Autodesk Inventor part; units mm, degrees
ref_plane "YZ Plane" through (0, 0, 0) normal (1, 0, 0) x (0, 1, 0)
ref_plane "XZ Plane" through (0, 0, 0) normal (0, 1, 0) x (-1, 0, 0)
ref_plane "XY Plane" through (0, 0, 0) normal (0, 0, 1) x (1, 0, 0)
sketch "Sketch1" plane through (0, 0, 0) normal (0, 0, 1) x (1, 0, 0)
  line L0 (0, 0) -> (38.1, 0)
  line L1 (38.1, 0) -> (48.2818, -36.7143)
  line L2 (38.1, 0) -> (76.2, 0) construction
  line L3 (45.343, 9.525) -> (9.525, 9.525)
  line L4 (0, 0) -> (0, 17.78)
  line L5 (0, 17.78) -> (9.525, 17.78)
  line L6 (9.525, 17.78) -> (9.525, 9.525)
  line L7 (0, 9.525) -> (9.525, 9.525)
  line L8 (45.343, 9.525) -> (38.1, 0)
  line L9 (48.2818, -36.7143) -> (69.6985, -30.7749)
  line L10 (69.6985, -30.7749) -> (67.153, -21.5964)
  line L11 (67.153, -21.5964) -> (54.9149, -24.9903)
  line L12 (54.9149, -24.9903) -> (45.343, 9.525)
  dimension "d0" = 38.1
  dimension "d1" = 38.1
  dimension "d2" = 74.5
  dimension "d9" = 17.78
  dimension "d10" = 9.525
  dimension "d11" = 9.525
  dimension "d12" = 22.225
  dimension "d13" = 9.525
  dimension "d14" = 12.7
extrude "Extrusion1" add sketch "Sketch1" along normal blind 10.16
properties part number "AttachmentPlateHopper_v3"
Work out the finished part from the listing and answer in its coordinate system (mm). A direction names the side the tool comes from. Coordinates: 2 decimals unless noted, no trailing zeros. Write each loop counter-clockwise with the first axis right and the second up, starting at its lowest first coordinate (ties: lowest second). Pieces come first, ordered by that corner, then holes. Notation, with made-up numbers: M 12.5,74 L 53.5,74 A12 cw 53.5,90 Z; hole C 11.5,14.5 d9. An arc over 180 degrees is marked long. Use one line per item in the form item = value. Start each with the question number.
1. The part is cut by section C-C (y = -26.5). Give the vertices of the cut face in (x, z).
2. The mould has two halves that part along X. Classify faces 4 (the face through (40, -3, 10.16)), 5 (the face through (43.12, -18.1, 5.01)), 6 (the face through (61.12, -23.27, 5.01)): released by +X, released by -X, zero draft, split by the parting line, or undercut.
3. The part is cut by section B-B (x = 8). Give the vertices of the cut face in (y, z), plus the area to 3 significant figures.
4. Straight lines are drawn through the part: probe 1 along Y at (x, z) = (28.5, 2.5) (3 decimals); probe 2 along X at (y, z) = (-5, 8); probe 3 along X at (y, z) = (-20.5, 5). For each, find the intervals that lie inside material, in ascending order. Write a range as from..to.
5. Each of these flat-tipped pins is pushed along its axis until it touches: P1, Ø2.5, axis at y = 15.5, z = 4, coming from the +X side (3 decimals); P2, Ø1.5, axis at x = 35, z = 9, coming from the -Y side. Where does it stop, or does it pass through?
6. The part is cut by section A-A (z = 4). Give the vertices of the cut face in (x, y) (1 decimal), plus the area to 3 significant figures.
7. A tool of negligible diameter and unlimited length cuts with its end or side. For faces 1 (the face through (19, 0, 5)), 2 (the face through (28, 9.525, 5)), 3 (the face through (0, 9, 5)), from which of +Z, -Z, +X, -X, +Y, -Y can it reach the whole face along a straight path? Write none if from no direction.
Evaluation:
q1.outline = M 45.45,0 L 68.51,0 L 68.51,10.16 L 45.45,10.16 Z
q2.face_4 = zero draft
q2.face_5 = released by -X
q2.face_6 = undercut
q3.outline = M 0,0 L 17.78,0 L 17.78,10.16 L 0,10.16 Z
q3.area = 181 mm^2
q4.probe_1 = 0..9.525
q4.probe_2 = 39.49..49.37
q4.probe_3 = 43.79..53.67
q5.P1 = 9.525
q5.P2 = 0
q6.outline = M 0,0 L 38.1,0 L 48.3,-36.7 L 69.7,-30.8 L 67.2,-21.6 L 54.9,-25 L 45.3,9.5 L 9.5,9.5 L 9.5,17.8 L 0,17.8 Z
q6.area = 994 mm^2
q7.face_1 = +Z, -Z, -X, -Y
q7.face_2 = +Z, -Z, +X, +Y
q7.face_3 = +Z, -Z, -X, +Y, -Y
